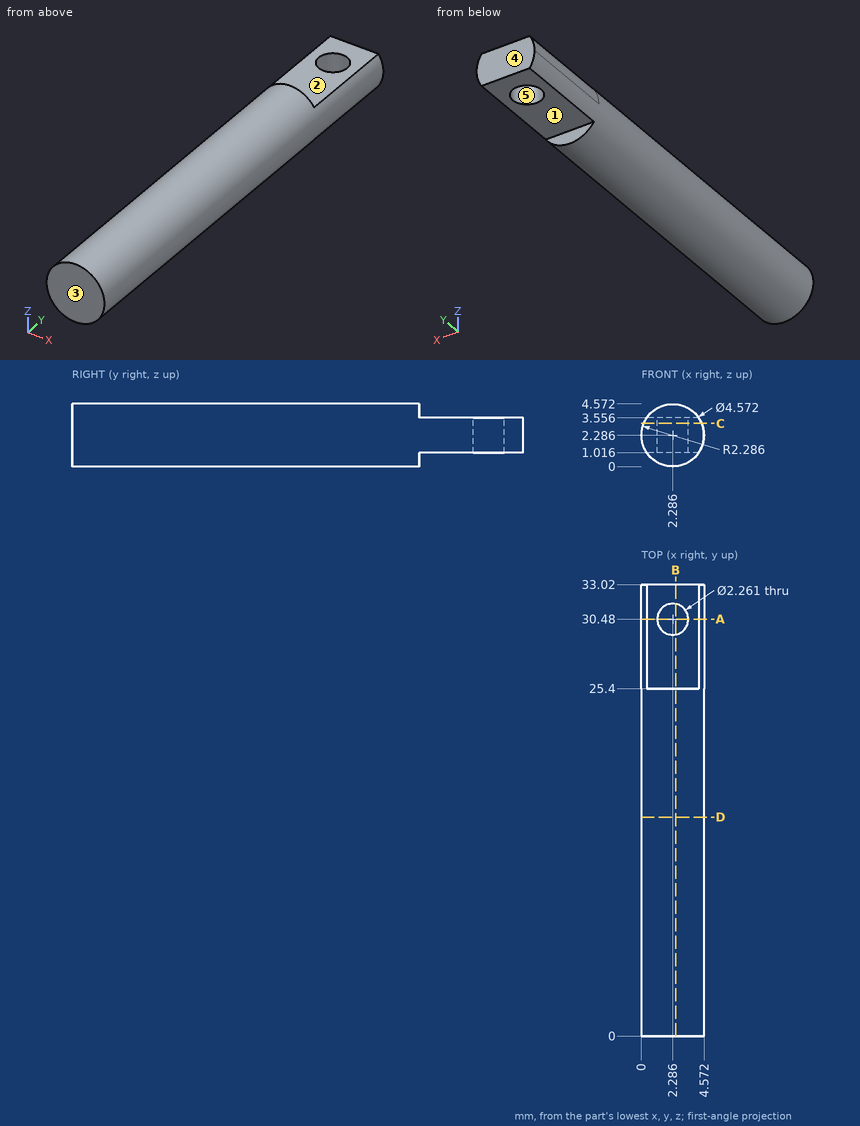
Geometry check sheet. Reference: drawing and pictorial views, mm from the part's lowest x, y, z. A direction names the side the tool comes from. Give positions to 0.01 mm unless a question says otherwise; leave off trailing zeros. Order: outer loops, then holes, each group sorted by start corner. A loop starts at its lowest first (then second) coordinate and runs counter-clockwise, first axis right, second up. Notation, with made-up numbers: M 35,80 L 62,80 A15 ccw 62,103 Z; hole C -38.5,75 d10. An arc over 180 degrees is marked long. Return JSON: item names as keys, results as strings. Group by question number.
1) Section check C-C on z = 3.15. Record the cut outline in (x, y), and give its area (3 significant figures).
2) Mould release check, pull along X, two halves, no side actions. Record for the marked faces 4 and 5: pulls with the +X half, pulls with the -X half, needs draft (parallel to the pull), parting line crosses it, or undercut.
3) Section check A-A on y = 30.48. Record the cut outline in (x, z) (1 decimal).
4) Access from +Z, -Z, +X, -X, +Y, -Y to the whole of each face (thin tool, end or side, straight path). Record for the marked faces 1, 2 and 3.
5) Section check D-D on y = 16. Record the cut outline in (x, z).
6) Section check B-B on x = 2.5. Record the cut outline in (y, z), and give its area (3 significant figures).
7) Scan lines: line 1 (Z direction, x = 2.15, y = 23); line 2 (Y direction, x = 1.85, z = 0.9); line 3 (Y direction, x = 2.05, z = 3) (1 decimal). Record each from-to range of solid material in increasing order.
8) Go/stop test with flat-tipped pins: pin 1 Ø0.8 at (x, z) = (2.5, 4) entering from +Y; pin 2 Ø1 at (y, z) = (26, 1.5) entering from +X; pin 3 Ø1 at (y, z) = (5.5, 4) entering from -X. Record where each tip stops, or that it passes through.
Answer block:
{
 "1": {"outline": "M 0.17,0 L 4.4,0 L 4.4,33.02 L 0.17,33.02 Z; hole C 2.29,30.48 d2.26", "area": "136 mm^2"},
 "2": {"face 4": "needs draft", "face 5": "undercut"},
 "3": {"outline": "M 0.4,1 L 1.2,1 L 1.2,3.6 L 0.4,3.6 A2.3 ccw Z; M 3.4,1 L 4.2,1 A2.3 ccw 4.2,3.6 L 3.4,3.6 Z"},
 "4": {"face 1": "-Z, +X, -X, +Y", "face 2": "+Z, +X, -X, +Y", "face 3": "+Z, -Z, +X, -X, -Y"},
 "5": {"outline": "C 2.29,2.29 d4.57"},
 "6": {"outline": "M 0,0.01 L 25.4,0.01 L 25.4,1.02 L 29.37,1.02 L 29.37,3.56 L 25.4,3.56 L 25.4,4.56 L 0,4.56 Z; M 31.59,1.02 L 33.02,1.02 L 33.02,3.56 L 31.59,3.56 Z", "area": "129 mm^2"},
 "7": {"line 1": "z = 0 to 4.57", "line 2": "y = 0 to 25.4", "line 3": "y = 0 to 29.4, 31.6 to 33"},
 "8": {"pin 1": "stops at y = 25.4", "pin 2": "stops at x = 4.55", "pin 3": "stops at x = 0.35"}
}
